Geometry: see drawing. Coordinates: mm, zero at the bounding-box minimum. A direction names the side the tool comes from. Coordinates: 2 decimals unless noted, no trailing zeros. Write each loop counter-clockwise with the first axis right and the second up, starting at its lowest first coordinate (ties: lowest second). Pieces come first, ordered by that corner, then holes.
1) Set-up query: the marked faces 1, 2 and 3. Return all of +Z, -Z, +X, -X, +Y, -Y with unobstructed straight access to the full face (end or side cutting, diameter ignored); none if empty.
2) Line query: L1, parallel to X at y = 11.5, z = 12.7; L2, parallel to Y at x = 6.35, z = 17.5; L3, parallel to Z at x = 6.5, y = 87. Output: solid intervals per line, ascending.
3) Draft query along X for the marked faces 4, 5 and 6. Return one class per face: pulls with the +X half, pulls with the -X half, needs draft (parallel to the pull), parting line crosses it, or undercut.
4) Section query C-C (x = 15). Output: boundary loops of the cut face in (y, z).
5) Pin query (flat end, axial travel): pin 1 Ø3 at (y, z) = (74, 13.5) entering from -X; pin 2 Ø3 at (x, y) = (6.35, 63.5) entering from -Z. Return the tip coordinate at first contact, or that it passes through.
6) Section query B-B (y = 47.5). State how many separate pieces and enclosed holes the cut face has, then the cut area to 3 significant figures.
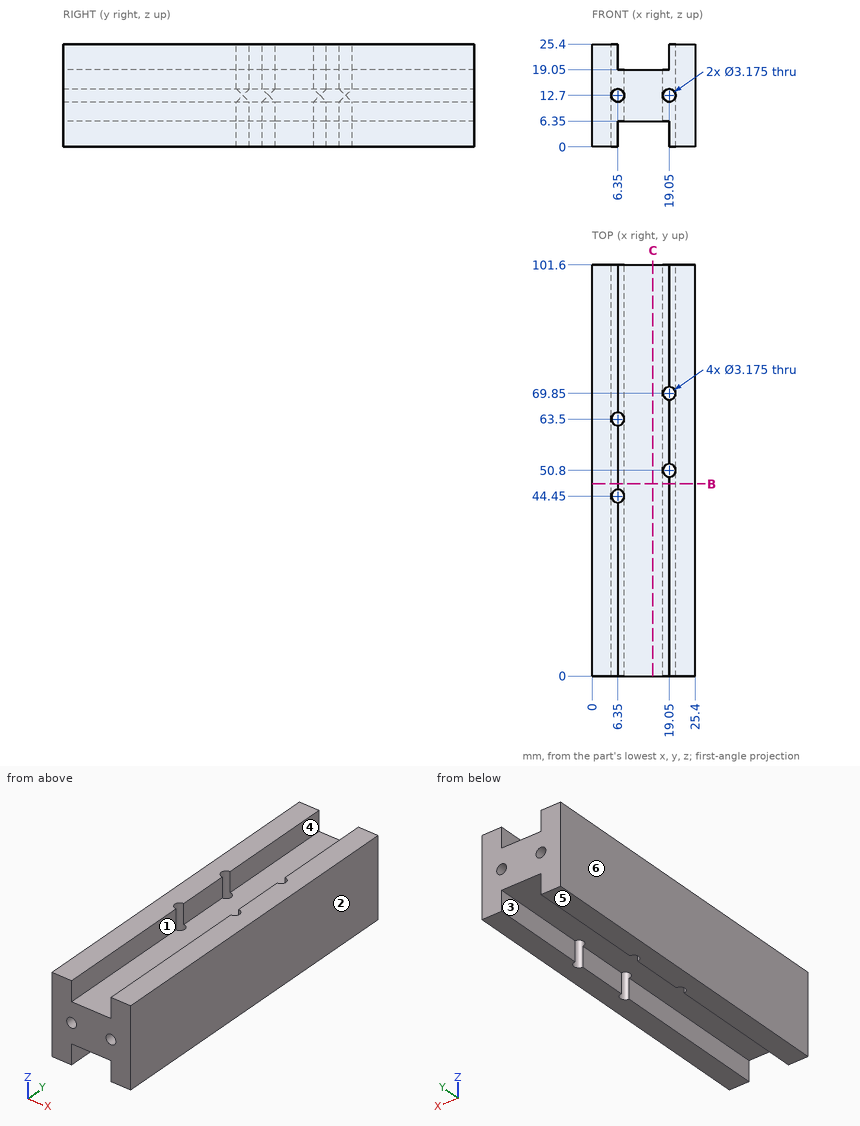
Answer:
1. face 1: +Z, +Y, -Y
1. face 2: +Z, -Z, +X, +Y, -Y
1. face 3: -Z, +Y, -Y
2. L1: x = 0 to 4.76, 7.94 to 17.46, 20.64 to 25.4
2. L2: y = 0 to 42.86, 46.04 to 61.91, 65.09 to 101.6
2. L3: z = 6.35 to 11.12, 14.28 to 19.05
3. face 4: undercut
3. face 5: needs draft
3. face 6: pulls with the -X half
4. outline: (0, 6.35) - (101.6, 6.35) - (101.6, 19.05) - (0, 19.05) - close
5. pin 1: stops at x = 0
5. pin 2: passes through
6. separate pieces: 1
6. enclosed holes: 2
6. area: 468 mm2
